Build history of the part. All positions in model axes, mm. A direction names the side the tool comes from. Coordinates: 2 decimals unless noted, no trailing zeros. Loops run counter-clockwise (first coordinate to the right, second up) from the corner with the lowest first, then second, coordinate; pieces in that order, holes last.
(1) Two-plate mould, pull along Y, no slides. Class faces 1 (the face through (0, 0, 0)), 2 (the face through (-2.994, 22.804, 10.437)), 3 (the face through (8.767, -16.856, 10.437)), 4 (the face through (0.325, -16.464, 2.958)): pulls with the +Y half, pulls with the -Y half, needs draft (parallel to the pull), parting line crosses it, or undercut.
(2) Slice it at B-B (y = -15). Give the cut face in (x, z), and give its area (3 significant figures).
(3) Flat gauge pins, fed straight in: P1, Ø1.5, axis at x = -5.5, z = 4, coming from the +Y side; P2, Ø1.5, axis at x = 3.5, z = 3.5, coming from the +Y side; P3, Ø1.8, axis at x = 0, y = -15, coming from the -Z side; P4, Ø1.5, axis at x = 7.5, z = 11, coming from the -Y side. Where does each tip first touch, or does it go through?
(4) Tool access for faces 5 (the face through (0, 0, 6)), 6 (the face through (3, 19, 15)): list every direction of +Z, -Z, +X, -X, +Y, -Y with a clear straight run to the whole face (end or side of a thin tool).
(5) Wall check: L1, parallel to X at y = 0, z = 12.5; L2, parallel to Z at x = 14, y = 7. Give the ranges that are in metal, low to high.
(6) Slice it at D-D (z = 1.5). Give the cut face in (x, y), and give its area (3 significant figures).
(7) Slice it at C-C (y = 0). Give the cut face in (x, z), and give its area (3 significant figures).
(8) Slice it at A-A (x = 0). Give the cut face in (y, z), and give its area (3 significant figures).
from build123d import *

# Parameters (mm, degrees)
SKETCH1_R           = 28
SKETCH1_R_2         = 23
SKETCH1_R_3         = 19
BOSS_EXTRUDE1_DEPTH = 6
SKETCH1_3_R         = 23
SKETCH1_3_R_2       = 19
BOSS_EXTRUDE2_DEPTH = 15
SKETCH2_R           = 1.5
CUT_EXTRUDE1_DEPTH  = 16


with BuildPart() as part:
    # Sketch1 → Boss-Extrude1 (new body)
    with BuildSketch(Plane.XY):
        Circle(SKETCH1_R)
        Circle(SKETCH1_R_2, mode=Mode.SUBTRACT)
        Circle(SKETCH1_R_2)
        Circle(SKETCH1_R_3, mode=Mode.SUBTRACT)
        Circle(SKETCH1_R_3)
    extrude(amount=BOSS_EXTRUDE1_DEPTH)

    # Sketch1_3 → Boss-Extrude2 (add)
    with BuildSketch(Plane.XY):
        Circle(SKETCH1_3_R)
        Circle(SKETCH1_3_R_2, mode=Mode.SUBTRACT)
    extrude(amount=BOSS_EXTRUDE2_DEPTH)

    # Sketch2 → Cut-Extrude1 (cut, through all)
    with BuildSketch(Plane(origin=(0, 0, 0), x_dir=(-1, 0, 0), z_dir=(0, 0, -1))):
        with Locations((0, -15)):
            Circle(SKETCH2_R)
    extrude(amount=-CUT_EXTRUDE1_DEPTH, mode=Mode.SUBTRACT)


solid = part.part
Response values:
1. face 1: needs draft
1. face 2: parting line crosses it
1. face 3: undercut
1. face 4: undercut
2. outline: (-23.64, 0) - (-1.5, 0) - (-1.5, 6) - (-11.66, 6) - (-11.66, 15) - (-17.44, 15) - (-17.44, 6) - (-23.64, 6) - close; (1.5, 0) - (23.64, 0) - (23.64, 6) - (17.44, 6) - (17.44, 15) - (11.66, 15) - (11.66, 6) - (1.5, 6) - close
2. area: 370 mm2
3. P1: stops at y = 27.59
3. P2: stops at y = 27.86
3. P3: passes through
3. P4: stops at y = -21.99
4. face 5: +Z
4. face 6: +Z, +X, -X, +Y, -Y
5. L1: x = -23 to -19, 19 to 23
5. L2: z = 0 to 6
6. outline: circle Ø56 at (0, 0); hole circle Ø3 at (0, -15)
6. area: 2,460 mm2
7. outline: (-28, 0) - (28, 0) - (28, 6) - (23, 6) - (23, 15) - (19, 15) - (19, 6) - (-19, 6) - (-19, 15) - (-23, 15) - (-23, 6) - (-28, 6) - close
7. area: 408 mm2
8. outline: (-28, 0) - (-16.5, 0) - (-16.5, 6) - (-19, 6) - (-19, 15) - (-23, 15) - (-23, 6) - (-28, 6) - close; (-13.5, 0) - (28, 0) - (28, 6) - (23, 6) - (23, 15) - (19, 15) - (19, 6) - (-13.5, 6) - close
8. area: 390 mm2
